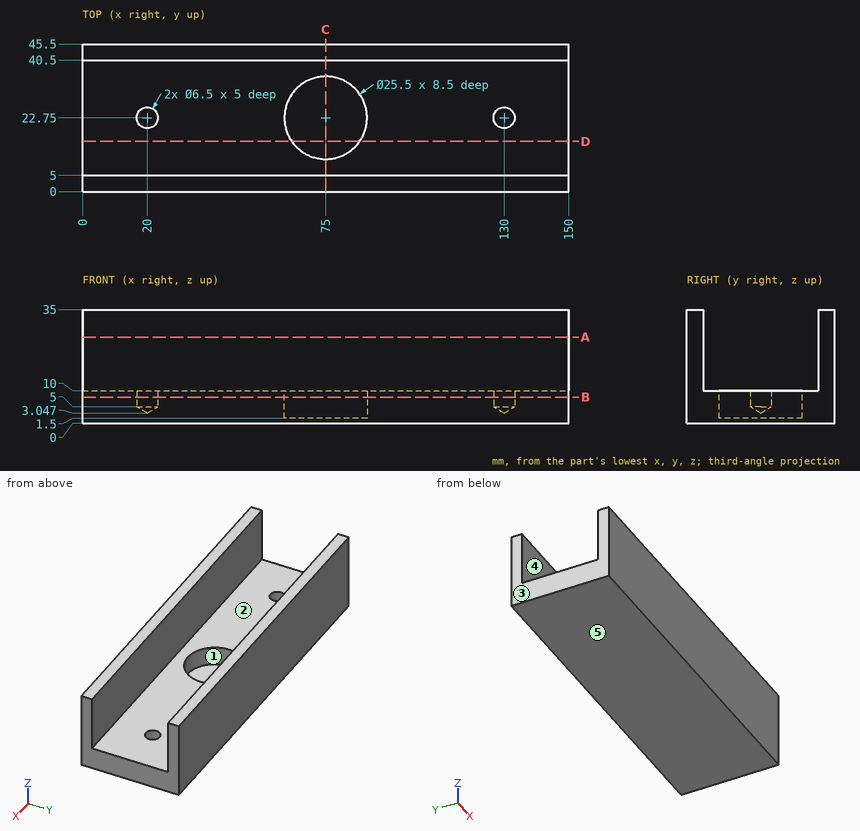
Could you check a few things on this drawing? It's one solid part, dimensions in mm from its lowest x, y, z. A direction names the side the tool comes from. Round coordinates to 2 decimals unless told otherwise and drop trailing zeros. Order: outer loops, then holes, each group sorted by start corner. A loop starts at its lowest first (then second) coordinate and runs counter-clockwise, first axis right, second up. Notation, with made-up numbers: (21.5, 63) -> (55.5, 63) arc R30 ccw to (55.5, 94) -> close; hole circle Ø2 at (70.25, -5.5). An arc over 180 degrees is marked (long way). One line per question, with ' | ' between items.
Q1. We'd pull the mould along X, two halves only. Please class the marked faces 1, 2 and 3: released by +X, released by -X, zero draft, split by the parting line, or undercut.
Computed values:
face 1: undercut | face 2: zero draft | face 3: released by -X
Q2. Which directions (+Z, -Z, +X, -X, +Y, -Y) give clear straight access to the entire face, cutting with the end or side of a thin tool? Please do the marked faces 4 and 5.
Computed values:
face 4: +Z, +X, -X | face 5: -Z, +X, -X, +Y, -Y
Q3. I'm going to push flat-ended pins straight in: pin 1 (5 mm diameter, centred on x = 27, z = 25, fed in from -Y); pin 2 (13 mm diameter, centred on x = 73.5, y = 22.5, fed in from +Z); pin 3 (6 mm diameter, centred on x = 20, y = 22.75, fed in from +Z); pin 4 (2 mm diameter, centred on x = 37.5, y = 34.5, fed in from +Z). Where does each tip first touch, or does it pass through?
Computed values:
pin 1: y = 0 | pin 2: z = 1.5 | pin 3: z = 4.85 | pin 4: z = 10
Q4. If we section it at B-B on z = 8: Write out the boundary of the cut face in (x, y), plus the area to 3 significant figures.
Computed values:
outline: (0, 0) -> (150, 0) -> (150, 45.5) -> (0, 45.5) -> close; hole circle Ø6.5 at (20, 22.75); hole circle Ø25.5 at (75, 22.75); hole circle Ø6.5 at (130, 22.75) | area: 6,250 mm²
Q5. If we section it at D-D on y = 15.5: Write out the boundary of the cut face in (x, z), plus the area to 3 significant figures.
Computed values:
outline: (0, 0) -> (150, 0) -> (150, 10) -> (85.49, 10) -> (85.49, 1.5) -> (64.51, 1.5) -> (64.51, 10) -> (0, 10) -> close | area: 1,320 mm²
Q6. If we section it at C-C on x = 75: Write out the boundary of the cut face in (y, z), plus the area to 3 significant figures.
Computed values:
outline: (0, 0) -> (45.5, 0) -> (45.5, 35) -> (40.5, 35) -> (40.5, 10) -> (35.5, 10) -> (35.5, 1.5) -> (10, 1.5) -> (10, 10) -> (5, 10) -> (5, 35) -> (0, 35) -> close | area: 488 mm²
Q7. If I drill on line 1 (Y direction, x = 20, z = 6); line 2 (Y direction, x = 134, z = 27.5); line 3 (X direction, y = 22, z = 8), over which ranges is the centre line in solid material (lowest first)? Write a range as from..to.
Computed values:
line 1: 0..19.5, 26..45.5 | line 2: 0..5, 40.5..45.5 | line 3: 0..16.84, 23.16..62.27, 87.73..126.84, 133.16..150
Q8. If we section it at A-A on z = 26.5: Write out the boundary of the cut face in (x, y).
Computed values:
outline: (0, 0) -> (150, 0) -> (150, 5) -> (0, 5) -> close; (0, 40.5) -> (150, 40.5) -> (150, 45.5) -> (0, 45.5) -> close
